Check sheet for the drawn part. Datum: minimum x, y, z corner. Units: mm. A direction names the side the tool comes from. Give positions to 0.01 mm unless a question says otherwise; leave off trailing zeros. Order: outer loops, then holes, each group sorted by start corner. A loop starts at its lowest first (then second) coordinate and runs counter-clockwise, first axis right, second up. Notation, with made-up numbers: (-24, 58) -> (26, 58) arc R31 ccw to (26, 87) -> close; hole circle Ø10 at (63, 17.5). An arc over 180 degrees is marked (long way). Answer in a Markdown table with one row per item. Add a question column.
(1) Cross-section at C-C (y = 4.25). Record the cut outline in (x, z).
(2) Thickness scan on L1, parallel to Z at x = 2.45, y = 12.75; L2, parallel to Z at x = 2.45, y = 10.5; L3, parallel to X at y = 18, z = 3.25. Record the ranges inside material, lowest first. Write a range as [from, to].
(3) Set-up check for the marked faces 4 and 5: record each of +Z, -Z, +X, -X, +Y, -Y from which the full face is reachable in a straight line by a thin tool's end or side.
(4) Cross-section at D-D (x = 3.4). Record the cut outline in (y, z).
(5) Cross-section at A-A (z = 2.45). Record the cut outline in (x, y), then the cut area to 4 significant figures.
(6) Go/stop test with flat-tipped pins: pin 1 (1.5 mm diameter, centred on y = 14.5, z = 4, fed in from +X); pin 2 (2.5 mm diameter, centred on x = 2.5, y = 14.5, fed in from -Z). Record where each tip stops, or that it passes through.
(7) Cross-section at B-B (x = 2.45). Record the cut outline in (y, z), then the cut area to 4 significant figures.
(8) Release check for a two-part mould opening along X. For the marked faces 1, 2 and 3 record: released by +X, released by -X, zero draft, split by the parting line, or undercut.
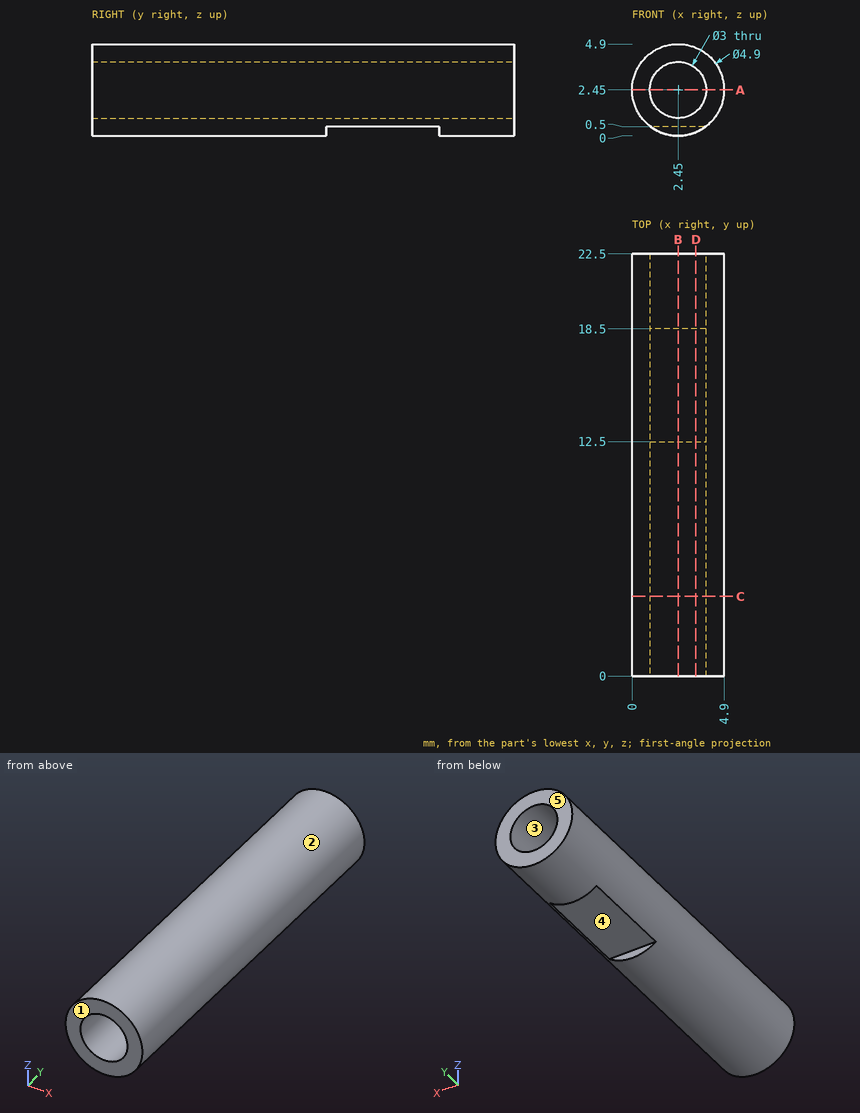
Answer below:
| question | item | result |
|---|---|---|
| 1 | outline | circle Ø4.9 at (2.45, 2.45); hole circle Ø3 at (2.45, 2.45) |
| 2 | L1 | z = [0.5, 0.95], [3.95, 4.9] |
| 2 | L2 | z = [0, 0.95], [3.95, 4.9] |
| 2 | L3 | x = [0.13, 1.18], [3.72, 4.77] |
| 3 | face 4 | -Z, +X, -X |
| 3 | face 5 | +Z, -Z, +X, -X, +Y |
| 4 | outline | (0, 0.19) -> (12.5, 0.19) -> (12.5, 0.5) -> (18.5, 0.5) -> (18.5, 0.19) -> (22.5, 0.19) -> (22.5, 1.29) -> (0, 1.29) -> close; (0, 3.61) -> (22.5, 3.61) -> (22.5, 4.71) -> (0, 4.71) -> close |
| 5 | outline | (0, 0) -> (0.95, 0) -> (0.95, 22.5) -> (0, 22.5) -> close; (3.95, 0) -> (4.9, 0) -> (4.9, 22.5) -> (3.95, 22.5) -> close |
| 5 | area | 42.75 mm² |
| 6 | pin 1 | stops at x = 4.77 |
| 6 | pin 2 | stops at z = 0.5 |
| 7 | outline | (0, 0) -> (12.5, 0) -> (12.5, 0.5) -> (18.5, 0.5) -> (18.5, 0) -> (22.5, 0) -> (22.5, 0.95) -> (0, 0.95) -> close; (0, 3.95) -> (22.5, 3.95) -> (22.5, 4.9) -> (0, 4.9) -> close |
| 7 | area | 39.75 mm² |
| 8 | face 1 | zero draft |
| 8 | face 2 | split by the parting line |
| 8 | face 3 | undercut |
